```python
from build123d import *

# Parameters (mm, degrees)
F0_R      = 8
F1_DEPTH  = 20.5
F2_W      = 16
F2_H      = 8
F3_DEPTH  = 13
F5_D      = 6
F8_D      = 5.2
F8_DEPTH  = 8
F8_START  = 0.434288
F8_TIP    = 1.5622376095
F9_R      = 8
F10_DEPTH = 2


with BuildPart() as f1:
    # F0 (on Top) → F1 (new body, symmetric)
    with BuildSketch(Plane.XY):
        Circle(F0_R)
    extrude(amount=F1_DEPTH, both=True)

    # F2 (on face) → F3 (cut)
    with BuildSketch(Plane(origin=(0, 0, -20.5), x_dir=(1, 0, 0), z_dir=(0, 0, -1))):
        with Locations((0, -4)):
            Rectangle(F2_W, F2_H)
    extrude(amount=-F3_DEPTH, mode=Mode.SUBTRACT)

    # F5 (through all)
    with Locations(Plane(origin=(0, 0, 0), x_dir=(-1, 0, 0), z_dir=(0, 1, 0))):
        with Locations((0, -14.5)):
            Hole(F5_D / 2)

    # F8
    # its depths count from where the whole tool has entered the part; down to there all is cleared
    with Locations(Plane(origin=(0, 8, 0), x_dir=(1, 0, 0), z_dir=(0, 1, 0)).offset(-F8_START)):
        with Locations((0, -14.5)):
            Hole(F8_D / 2, depth=F8_DEPTH)
            with Locations((0, 0, -(F8_DEPTH + F8_TIP / 2))):  # 118° drill point
                Cone(0, F8_D / 2, F8_TIP, mode=Mode.SUBTRACT)

    # F9 (on face) → F10 (cut)
    with BuildSketch(Plane.XY.offset(20.5)):
        Circle(F9_R)
    extrude(amount=-F10_DEPTH, mode=Mode.SUBTRACT)


solid = f1.part
```
Model file for the job. Use its own axes, mm. A direction names the side the tool comes from. Round coordinates to 2 decimals unless told otherwise and drop trailing zeros. Write each loop counter-clockwise with the first axis right and the second up, starting at its lowest first coordinate (ties: lowest second). Pieces come first, ordered by that corner, then holes. Notation, with made-up numbers: M 26,41 L 75,41 A12 ccw 75,46 Z; hole C 58.5,-6 d11. An arc over 180 degrees is marked long. Put each result on its own line as item: value.
Item 1: Probe L1, parallel to Z at x = 0, y = 2; L2, parallel to Z at x = 0, y = -6; L3, parallel to X at y = -4, z = -12. List the from-to ranges inside material, lowest first. Write a range as from..to.
Responses:
L1: -7.5..11.9, 17.1..18.5
L2: -20.5..-17.5, -11.5..18.5
L3: -6.93..-1.66, 1.66..6.93
Item 2: Cut at A-A (z = -14.5). List the corners of the cut face in (x, y), and give its area (3 significant figures).
Responses:
outline: M -8,0 A8 ccw -3,-7.42 L -3,0 Z; M 3,-7.42 A8 ccw 8,0 L 3,0 Z
area: 53.7 mm²
Item 3: Mould opens along X. For faces 1 (the cylindrical face through (3.69, -7.1, 3.61)), 2 (the cylindrical face through (0.56, 3.73, 17.04)), 3 (the flat face through (0, 0, 18.5)) say: +X half, -X half, draft (parallel to the pull), parting line (faces both ways), or undercut.
Responses:
face 1: parting line
face 2: undercut
face 3: draft
Item 4: Cut at C-C (x = -4.75). List the corners of the cut face in (y, z), and give its area (3 significant figures).
Responses:
outline: M -6.44,-20.5 L 0,-20.5 L 0,-7.5 L 6.44,-7.5 L 6.44,18.5 L -6.44,18.5 Z
area: 418 mm²
Item 5: Cut at B-B (y = 5.5). List the corners of the cut face in (x, z), and give its area (3 significant figures).
Responses:
outline: M -5.81,-7.5 L 5.81,-7.5 L 5.81,18.5 L -5.81,18.5 Z; hole C 0,14.5 d5.2
area: 281 mm²
Item 6: Cut at D-D (y = -6.5). List the corners of the cut face in (x, z), and give its area (3 significant figures).
Responses:
outline: M -4.66,-20.5 L 4.66,-20.5 L 4.66,18.5 L -4.66,18.5 Z; hole C 0,-14.5 d6
area: 335 mm²
Item 7: Tool access for faces 4 (the flat face through (0, -3, -20.5)), 5 (the flat face through (0, 3, -7.5)): list every direction of +Z, -Z, +X, -X, +Y, -Y with a clear straight run to the whole face (end or side of a thin tool).
Responses:
face 4: -Z, +X, -X, +Y, -Y
face 5: -Z, +X, -X, +Y
Item 8: Flat gauge pins, fed straight in: P1, Ø7, axis at x = 0, z = -14.5, coming from the +Y side; P2, Ø1.5, axis at x = -3, y = 5, coming from the -Z side; P3, Ø6, axis at y = -5, z = -4.5, coming from the +X side. Where does each tip first touch, or does it go through?
Responses:
P1: y = 0
P2: z = -7.5
P3: x = 7.75
